from build123d import *

# Parameters (mm, degrees)
F1_W     = 70
F1_H     = 45
F2_DEPTH = 5
F3_R     = 1.508
F4_DEPTH = 25
F5_R     = 3.0876875
F6_DEPTH = 25
F7_R     = 5.921375
F8_DEPTH = 1.5875


# Not quite as in the source:
# - a length typed as a fraction of an inch, garbled in the dataset ("3 / 203.2 mm" for 3/8 in), is restored


with BuildPart() as f2:
    # F1 (on Top) → F2 (new body)
    with BuildSketch(Plane.XY):
        with Locations((-0.7, 0)):
            Rectangle(F1_W, F1_H)
    extrude(amount=-F2_DEPTH)

    # F3 (on Top) → F4 (cut)
    with BuildSketch(Plane.XY):
        with Locations((-25.3, 0)):
            Circle(F3_R)
        with Locations((22.04, 15.9)):
            Circle(F3_R)
        with Locations((22.04, -15.9)):
            Circle(F3_R)
    extrude(amount=-F4_DEPTH, mode=Mode.SUBTRACT)

    # F5 (on Top) → F6 (cut)
    with BuildSketch(Plane.XY):
        with Locations((-8.2, 7.5)):
            Circle(F5_R)
        with Locations((6.8, 7.5)):
            Circle(F5_R)
        with Locations((-8.2, -7.5)):
            Circle(F5_R)
        with Locations((6.8, -7.5)):
            Circle(F5_R)
    extrude(amount=-F6_DEPTH, mode=Mode.SUBTRACT)

    # F7 (on face) → F8 (cut)
    with BuildSketch(Plane.XY):
        with Locations((-8.2, 7.5)):
            Circle(F7_R)
        with Locations((6.8, 7.5)):
            Circle(F7_R)
        with Locations((-8.2, -7.5)):
            Circle(F7_R)
        with Locations((6.8, -7.5)):
            Circle(F7_R)
    extrude(amount=-F8_DEPTH, mode=Mode.SUBTRACT)


solid = f2.part
Can you work these out from the model? Positions are in its coordinate system, mm. A direction names the side the tool comes from. Give positions to 0.01 mm unless a question says otherwise; leave off trailing zeros. Loops run counter-clockwise (first coordinate to the right, second up) from the corner with the lowest first, then second, coordinate; pieces in that order, holes last. Notation, with made-up numbers: M -29,39.25 L 13,39.25 A21 cw 13,46.25 Z; hole C -26,20 d8. An arc over 180 degrees is marked long. One line per item, written item: value.
1) Imagine slicing it at C-C on z = -0.9. Write out the boundary of the cut face in (x, y), and give its area (3 significant figures).
Geometry check:
outline: M -35.7,-22.5 L 34.3,-22.5 L 34.3,22.5 L -35.7,22.5 Z; hole C -25.3,0 d3.02; hole C -8.2,-7.5 d11.84; hole C -8.2,7.5 d11.84; hole C 6.8,-7.5 d11.84; hole C 6.8,7.5 d11.84; hole C 22.04,-15.9 d3.02; hole C 22.04,15.9 d3.02
area: 2,690 mm²
2) Please list where these lines run through material, in increasing order: line 1 (Y direction, x = 6.8, z = -0.8); line 2 (X direction, y = 16, z = -1); line 3 (X direction, y = 10, z = -4.35).
Geometry check:
line 1: y = -22.5 to -13.42, -1.58 to 1.58, 13.42 to 22.5
line 2: x = -35.7 to 20.54, 23.54 to 34.3
line 3: x = -35.7 to -10.01, -6.39 to 4.99, 8.61 to 34.3
3) I'm going to push flat-ended pins straight in: pin 1 (2.5 mm diameter, centred on x = -25.3, y = 0, fed in from +Z); pin 2 (10 mm diameter, centred on x = 0, y = -4.5, fed in from +Z); pin 3 (9.5 mm diameter, centred on x = 6.8, y = 7.5, fed in from +Z). Where does each tip first touch, or does it pass through?
Geometry check:
pin 1: passes through
pin 2: stops at z = 0
pin 3: stops at z = -1.59
4) On a 3-axis mill with a long thin cutter (end or side, diameter ignored), from which of +Z, -Z, +X, -X, +Y, -Y can I reach the whole of each face in a straight line? I mean faces 4 (the face through (12.448, -5.721, -0.783)), 5 (the face through (23.48, 16.35, -2.46)). Say none if no direction works.
Geometry check:
face 4: +Z
face 5: +Z, -Z
5) Imagine slicing it at A-A on y = -15.9. Write out the boundary of the cut face in (x, z), and give its area (3 significant figures).
Geometry check:
outline: M -35.7,-5 L 20.53,-5 L 20.53,0 L -35.7,0 Z; M 23.55,-5 L 34.3,-5 L 34.3,0 L 23.55,0 Z
area: 335 mm²
6) Thinking about a two-plate mould opening in X: for faces 1 (the face through (-1, 0, 0)), 2 (the face through (-10.476, -5.413, -3.27)), 3 (the face through (34.3, 0, -2)), which applies, +X half, -X half, draft (parallel to the pull), parting line (faces both ways), or undercut?
Geometry check:
face 1: draft
face 2: undercut
face 3: +X half
7) Imagine slicing it at D-D on y = -7.5. Write out the boundary of the cut face in (x, z).
Geometry check:
outline: M -35.7,-5 L -11.29,-5 L -11.29,-1.59 L -14.12,-1.59 L -14.12,0 L -35.7,0 Z; M -5.11,-5 L 3.71,-5 L 3.71,-1.59 L 0.88,-1.59 L 0.88,0 L -2.28,0 L -2.28,-1.59 L -5.11,-1.59 Z; M 9.89,-5 L 34.3,-5 L 34.3,0 L 12.72,0 L 12.72,-1.59 L 9.89,-1.59 Z
8) Imagine slicing it at B-B on x = -25.3. Write out the boundary of the cut face in (y, z), and give its area (3 significant figures).
Geometry check:
outline: M -22.5,-5 L -1.51,-5 L -1.51,0 L -22.5,0 Z; M 1.51,-5 L 22.5,-5 L 22.5,0 L 1.51,0 Z
area: 210 mm²
